Part print with two shaded views. Sizes in mm from the minimum x, y, z corner. A direction names the side the tool comes from. Round coordinates to 2 decimals unless told otherwise and drop trailing zeros. Loops run counter-clockwise (first coordinate to the right, second up) from the corner with the lowest first, then second, coordinate; pieces in that order, holes last. Notation, with made-up numbers: M -26.5,9 L 5.5,9 A30 cw 5.5,43 Z; hole C 36,25 d9. An arc over 180 degrees is marked long. Put each result on its own line as item: value. Start each with the question number.
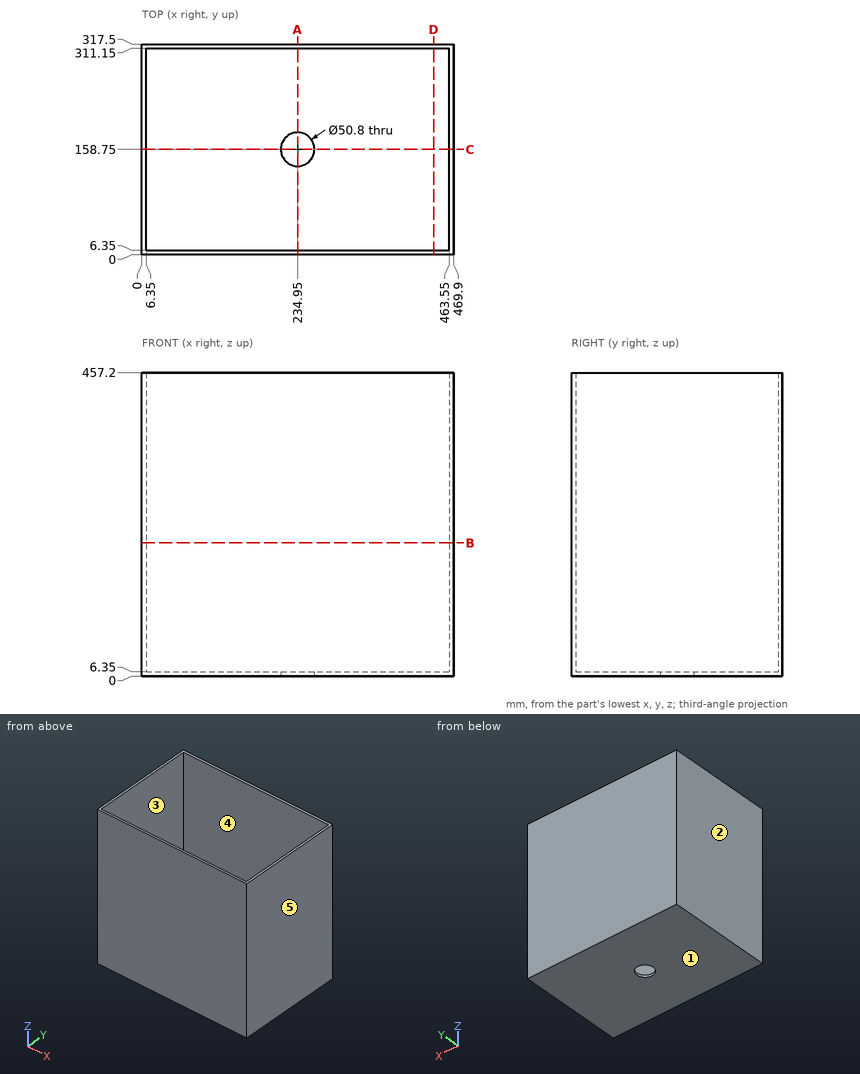
(1) Cut at C-C on y = 158.75. List the corners of the cut face in (x, z), and give its area (3 significant figures).
(2) Tool access for the marked faces 4 and 5: list every direction of +Z, -Z, +X, -X, +Y, -Y with a clear straight run to the whole face (end or side of a thin tool).
(3) Flat gauge pins, fed straight in: pin 1 Ø1.5 at (x, y) = (110.5, 98) entering from +Z; pin 2 Ø12 at (x, y) = (291.5, 136.5) entering from -Z. Where does each tip first touch, or does it go through?
(4) Cut at D-D on x = 440. List the corners of the cut face in (y, z).
(5) Cut at B-B on z = 200.5. List the corners of the cut face in (x, y).
(6) Drill centre lines: line 1 along Y through (x, z) = (234, 2); line 2 along Y through (x, z) = (91, 260.5); line 3 along X through (y, z) = (231.5, 420). Where is each one in solid material? Low to high.
(7) Mould opens along X. For the marked faces 1, 2 and 3 say: +X half, -X half, draft (parallel to the pull), parting line (faces both ways), or undercut.
(8) Cut at A-A on x = 234.95. List the corners of the cut face in (y, z), and give its area (3 significant figures).
Taken from the geometry:
1. outline: M 0,0 L 209.55,0 L 209.55,6.35 L 6.35,6.35 L 6.35,457.2 L 0,457.2 Z; M 260.35,0 L 469.9,0 L 469.9,457.2 L 463.55,457.2 L 463.55,6.35 L 260.35,6.35 Z
1. area: 8,390 mm2
2. face 4: +Z
2. face 5: +Z, -Z, +X, +Y, -Y
3. pin 1: z = 6.35
3. pin 2: z = 0
4. outline: M 0,0 L 317.5,0 L 317.5,457.2 L 311.15,457.2 L 311.15,6.35 L 6.35,6.35 L 6.35,457.2 L 0,457.2 Z
5. outline: M 0,0 L 469.9,0 L 469.9,317.5 L 0,317.5 Z; hole M 6.35,6.35 L 463.55,6.35 L 463.55,311.15 L 6.35,311.15 Z
6. line 1: 0 to 133.37, 184.13 to 317.5
6. line 2: 0 to 6.35, 311.15 to 317.5
6. line 3: 0 to 6.35, 463.55 to 469.9
7. face 1: draft
7. face 2: -X half
7. face 3: undercut
8. outline: M 0,0 L 133.35,0 L 133.35,6.35 L 6.35,6.35 L 6.35,457.2 L 0,457.2 Z; M 184.15,0 L 317.5,0 L 317.5,457.2 L 311.15,457.2 L 311.15,6.35 L 184.15,6.35 Z
8. area: 7,420 mm2
